For this review, take the finished solid that the model builds, in its own axes (mm). Face numbers are marked on the shaded views. A direction names the side the tool comes from. Give positions to 0.01 mm unless a question says otherwise; leave off trailing zeros. Write each loop counter-clockwise with the first axis right and the second up, starting at its lowest first coordinate (ties: lowest second). Pieces come first, ordered by that corner, then holes. Notation, with made-up numbers: M -24.75,19.5 L 13.25,19.5 A21 cw 13.25,38.5 Z; hole C -19.75,-35.5 d3. An arc over 180 degrees is marked long. One line per item, written item: value. Start each with the question number.
Item 1: Consider section A-A, the plane z = -5. Write out the cut boundary in (x, y), and give its area (3 significant figures).
Item 2: To check wall thickness, follow probe 1 along Z at (x, y) = (5.5, 0.8); probe 2 along Z at (x, y) = (5.5, 3.6); probe 3 along X at (y, z) = (14, -10.75). State the ranges of each line that lie inside material, in increasing order.
Item 3: Consider section B-B, the plane x = 5.5. Write out the cut boundary in (y, z).
Item 4: Mouldability with a two-part tool opening along Y and no side actions: class the marked faces 5, 6, 7 and 8 as released by +Y, released by -Y, zero draft, split by the parting line, or undercut.
Item 5: Tool access review of the marked faces 1, 2, 3 and 4: name each direction out of +Z, -Z, +X, -X, +Y, -Y from which nothing blocks a thin tool from reaching the whole face with its end or side.
Item 6: Consider section D-D, the plane y = 15.5. Write out the cut boundary in (x, z).
Item 7: Consider section C-C, the plane z = 0. Write out the cut boundary in (x, y).
Item 8: Clearance check with flat-ended pins moving along their axes: pin 1 Ø13 at (x, z) = (5.5, 0) entering from -Y; pin 2 Ø4 at (x, z) = (5, 1.5) entering from +Y; pin 3 Ø4 at (x, y) = (6, 3.5) entering from +Z; pin 4 Ø7.5 at (x, z) = (9.5, -2.5) entering from +Y. State where each tip first meets the part, or that it passes through.
Autodesk Inventor part; units mm, degrees
ref_plane "YZ Plane" through (0, 0, 0) normal (1, 0, 0) x (0, 1, 0)
ref_plane "XZ Plane" through (0, 0, 0) normal (0, 1, 0) x (-1, 0, 0)
ref_plane "XY Plane" through (0, 0, 0) normal (0, 0, 1) x (1, 0, 0)
sketch "Sketch1" plane through (0, 0, 0) normal (0, 1, 0) x (-1, 0, 0)
  line L0 (-17.5, -12.5) -> (17.5, -12.5)
  line L1 (17.5, -12.5) -> (17.5, 12.5)
  line L2 (17.5, 12.5) -> (-17.5, 12.5)
  line L3 (-17.5, 12.5) -> (-17.5, -12.5)
  line L4 (-17.5, -12.5) -> (17.5, 12.5) construction
  line L5 (17.5, -12.5) -> (-17.5, 12.5) construction
  line L6 (-17.5, 0) -> (17.5, 0) construction
  line L7 (0.5, 12.5) -> (0.5, 9.5)
  line L8 (0.5, 9.5) -> (-11.5, 9.5)
  line L9 (-11.5, 9.5) -> (-11.5, 12.5)
  line L10 (-11.5, 15.5) -> (0.5, 9.5) construction
  line L11 (0.5, 15.5) -> (-11.5, 9.5) construction
  line L12 (0.5, -12.5) -> (0.5, -9.5)
  line L13 (0.5, -9.5) -> (-11.5, -9.5)
  line L14 (-11.5, -9.5) -> (-11.5, -12.5)
  circle A0 centre (-5.5, 0) radius 4
  point P0 (0, 0)
  point P1 (-5.5, 12.5)
  dimension "d0" = 35
  dimension "d1" = 25
  dimension "d2" = 6
  dimension "d3" = 12
  dimension "d4" = 6
  dimension "d5" = 19
  dimension "d6" = 8
extrude "Extrusion1" add sketch "Sketch1" along normal blind 5 contours L3 L2 L9 L8 L7 L1 L0 L12 L13 L14
sketch "Sketch2" plane through (-17.5, 0, -12.5) normal (-1, 0, 0) x (0, 0, 1)
  line L0 (22, 0) -> (25, 0)
  line L1 (0, 0) -> (25, 0)
  line L2 (25, 0) -> (25, 18)
  line L3 (25, 18) -> (0, 18)
  line L4 (0, 18) -> (0, 0)
  point P0 (12.5, 0)
  dimension "d9" = 18
  dimension "d10" = 25
extrude "Extrusion2" add sketch "Sketch2" against normal blind 5
sketch "Sketch3" plane through (-17.5, 0, -12.5) normal (-1, 0, 0) x (0, 0, 1)
  line L0 (5, 13) -> (20, 13) construction
  line L1 (5, 10) -> (20, 10)
  line L2 (20, 16) -> (5, 16)
  arc A0 (5, 16) -> (5, 10) centre (5, 13) ccw
  arc A1 (20, 10) -> (20, 16) centre (20, 13) ccw
  line L3 (0, 0) -> (0, 18)
  line L4 (25, 18) -> (0, 18)
  point P0 (12.5, 0)
  point P1 (12.5, 13)
  dimension "d16" = 12.5
  dimension "d17" = 15
  dimension "d18" = 5
  dimension "d19" = 3
extrude "Extrusion3" cut sketch "Sketch3" against normal blind 5
sketch "Sketch4" plane through (0, 0, 0) normal (0, 1, 0) x (-1, 0, 0)
  circle A0 centre (-5.5, 0) radius 4
  circle A1 centre (-5.5, 0) radius 2.5
  point P0 (0, 0)
  dimension "d22" = 5
extrude "Extrusion4" add sketch "Sketch4" along normal blind 3
fillet "Fillet1" radius 5 2 edges at (-15, 18, 12.5) (-15, 18, -12.5)
fillet "Fillet2" radius 2 1 edges at (-12.5, 5, 0)
fillet "Fillet3" radius 4 2 edges at (17.5, 2.5, 12.5) (17.5, 2.5, -12.5)
properties part number "ejercicio 266" material "Thermoplastic Resin"
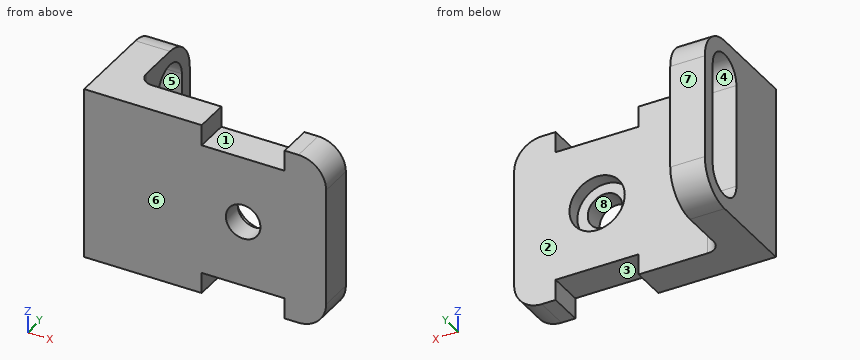
Model answer:
1. outline: M -17.5,0 L 17.5,0 L 17.5,5 L -10.5,5 A2 cw -12.5,7 L -12.5,10 L -17.5,10 Z; M -17.5,16 L -12.5,16 L -12.5,18 L -17.5,18 Z
1. area: 211 mm2
2. probe 1: z = -9.5 to -2.5, 2.5 to 9.5
2. probe 2: z = -9.5 to -4, 4 to 9.5
2. probe 3: x = -17.5 to -12.5
3. outline: M 0,-9.5 L 5,-9.5 L 5,-4 L 3,-4 L 3,-2.5 L 0,-2.5 Z; M 0,2.5 L 3,2.5 L 3,4 L 5,4 L 5,9.5 L 0,9.5 Z
4. face 5: undercut
4. face 6: released by -Y
4. face 7: released by +Y
4. face 8: zero draft
5. face 1: +Z, +Y, -Y
5. face 2: +Z, -Z, +X, +Y
5. face 3: -Z, +Y, -Y
5. face 4: +X, -X
6. outline: M -17.5,-11.83 L -12.5,-11.83 L -12.5,-9.16 L -17.5,-9.16 Z; M -17.5,9.16 L -12.5,9.16 L -12.5,11.83 L -17.5,11.83 Z
7. outline: M -17.5,0 L 3,0 L 3,3 L 1.5,3 L 1.5,5 L -10.5,5 A2 cw -12.5,7 L -12.5,10 L -17.5,10 Z; M -17.5,16 L -12.5,16 L -12.5,18 L -17.5,18 Z; M 8,0 L 17.5,0 L 17.5,5 L 9.5,5 L 9.5,3 L 8,3 Z
8. pin 1: stops at y = 0
8. pin 2: stops at y = 3
8. pin 3: stops at z = 9.5
8. pin 4: stops at y = 5
